Geometry check sheet. Reference: the model listing, model coordinates, mm. Coordinates: 2 decimals unless noted, no trailing zeros. Loops run counter-clockwise (first coordinate to the right, second up) from the corner with the lowest first, then second, coordinate; pieces in that order, holes last.
from build123d import *

# Parameters (mm, degrees)
SKETCH_1_R      = 140
SKETCH_1_R_2    = 8.5
EXTRUDE_1_DEPTH = 5


with BuildPart() as part:
    # ｽｹｯﾁ1 → ﾎﾞｽ - 押し出し1 (new body)
    with BuildSketch(Plane(origin=(0, 0, 0), x_dir=(1, 0, 0), z_dir=(0, 1, 0))):
        with Locations(Location((0, 0, 0), (0, 0, 270))):
            Circle(SKETCH_1_R)
        with Locations(Location((0, 0, 0), (0, 0, 270))):
            Circle(SKETCH_1_R_2, mode=Mode.SUBTRACT)
        with BuildLine():
            Line((-108.166538264, 10), (-32.897568299, 10))
            ThreePointArc((-32.897568299, 10), (-27.995938568, 11.283691953), (-24.352745364, 14.805194805))
            ThreePointArc((-24.352745364, 14.805194805), (-20.152543264, 20.152543264), (-14.805194805, 24.352745364))
            ThreePointArc((-14.805194805, 24.352745364), (-11.283691953, 27.995938568), (-10, 32.897568299))
            Line((-10, 32.897568299), (-10, 108.166538264))
            ThreePointArc((-10, 108.166538264), (-13.603978509, 115.853599412), (-21.818181818, 117.999859924))
            ThreePointArc((-21.818181818, 117.999859924), (-84.852813742, 84.852813742), (-117.999859924, 21.818181818))
            ThreePointArc((-117.999859924, 21.818181818), (-115.853599412, 13.603978509), (-108.166538264, 10))
        make_face(mode=Mode.SUBTRACT)
        with BuildLine():
            Line((10, 108.166538264), (10, 32.897568299))
            ThreePointArc((10, 32.897568299), (11.283691953, 27.995938568), (14.805194805, 24.352745364))
            ThreePointArc((14.805194805, 24.352745364), (20.152543264, 20.152543264), (24.352745364, 14.805194805))
            ThreePointArc((24.352745364, 14.805194805), (27.995938568, 11.283691953), (32.897568299, 10))
            Line((32.897568299, 10), (108.166538264, 10))
            ThreePointArc((108.166538264, 10), (115.853599412, 13.603978509), (117.999859924, 21.818181818))
            ThreePointArc((117.999859924, 21.818181818), (84.852813742, 84.852813742), (21.818181818, 117.999859924))
            ThreePointArc((21.818181818, 117.999859924), (13.603978509, 115.853599412), (10, 108.166538264))
        make_face(mode=Mode.SUBTRACT)
        with BuildLine():
            Line((108.166538264, -10), (32.897568299, -10))
            ThreePointArc((32.897568299, -10), (27.995938568, -11.283691953), (24.352745364, -14.805194805))
            ThreePointArc((24.352745364, -14.805194805), (20.152543264, -20.152543264), (14.805194805, -24.352745364))
            ThreePointArc((14.805194805, -24.352745364), (11.283691953, -27.995938568), (10, -32.897568299))
            Line((10, -32.897568299), (10, -108.166538264))
            ThreePointArc((10, -108.166538264), (13.603978509, -115.853599412), (21.818181818, -117.999859924))
            ThreePointArc((21.818181818, -117.999859924), (84.852813742, -84.852813742), (117.999859924, -21.818181818))
            ThreePointArc((117.999859924, -21.818181818), (115.853599412, -13.603978509), (108.166538264, -10))
        make_face(mode=Mode.SUBTRACT)
        with BuildLine():
            Line((-10, -108.166538264), (-10, -32.897568299))
            ThreePointArc((-10, -32.897568299), (-11.283691953, -27.995938568), (-14.805194805, -24.352745364))
            ThreePointArc((-14.805194805, -24.352745364), (-20.152543264, -20.152543264), (-24.352745364, -14.805194805))
            ThreePointArc((-24.352745364, -14.805194805), (-27.995938568, -11.283691953), (-32.897568299, -10))
            Line((-32.897568299, -10), (-108.166538264, -10))
            ThreePointArc((-108.166538264, -10), (-115.853599412, -13.603978509), (-117.999859924, -21.818181818))
            ThreePointArc((-117.999859924, -21.818181818), (-84.852813742, -84.852813742), (-21.818181818, -117.999859924))
            ThreePointArc((-21.818181818, -117.999859924), (-13.603978509, -115.853599412), (-10, -108.166538264))
        make_face(mode=Mode.SUBTRACT)
    extrude(amount=EXTRUDE_1_DEPTH)


solid = part.part
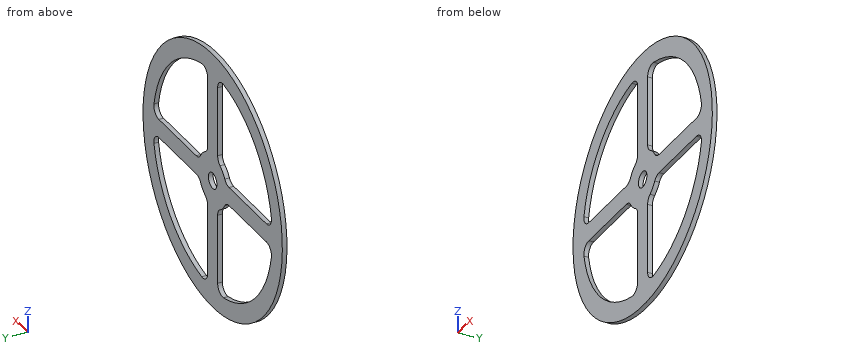
(1) Sectioned sample at B-B on y = 3.35. State how many separate pieces and enclosed holes the cut face has, and give its area (3 significant figures).
Findings:
separate pieces: 1
enclosed holes: 5
area: 26,300 mm2
(2) Scan lines: L1, parallel to Z at x = -66, y = 0.2; L2, parallel to Z at x = -20.5, y = 3.95; L3, parallel to X at y = 4.3, z = -69.5. Record each from-to range of solid material in increasing order.
Findings:
L1: z = -123.47 to -100.22, -10 to 10, 100.22 to 123.47
L2: z = -138.49 to -118.15, -19.8 to 19.8, 118.15 to 138.49
L3: x = -121.53 to -97.83, -10 to 10, 97.83 to 121.53
(3) Sectioned sample at A-A on z = 0. Record the cut outline in (x, y), and give its area (4 significant figures).
Findings:
outline: (-140, 0) - (-8.5, 0) - (-8.5, 5) - (-140, 5) - close; (8.5, 0) - (140, 0) - (140, 5) - (8.5, 5) - close
area: 1,315 mm2
(4) Gauge pin test, flat ends, axial feed: pin 1 Ø12 at (x, z) = (-95, 10) entering from -Y; pin 2 Ø1.5 at (x, y) = (-88.5, 3.5) entering from -Z; pin 3 Ø1 at (x, y) = (-27.5, 3) entering from +Z; pin 4 Ø1.5 at (y, z) = (3.5, 67) entering from -X. Record the tip position at first contact, or that the pin passes through.
Findings:
pin 1: stops at y = 0
pin 2: stops at z = -109.09
pin 3: stops at z = 137.37
pin 4: stops at x = -123.33
(5) Sectioned sample at D-D on z = 75. Record the cut outline in (x, y).
Findings:
outline: (-118.22, 0) - (-93.67, 0) - (-93.67, 5) - (-118.22, 5) - close; (-10, 0) - (10, 0) - (10, 5) - (-10, 5) - close; (93.67, 0) - (118.22, 0) - (118.22, 5) - (93.67, 5) - close
(6) Sectioned sample at C-C on x = 0. Record the cut outline in (y, z).
Findings:
outline: (0, -140) - (5, -140) - (5, -8.5) - (0, -8.5) - close; (0, 8.5) - (5, 8.5) - (5, 140) - (0, 140) - close
